from build123d import *

# Parameters (mm, degrees)
SKETCH2_W               = 20
SKETCH2_H               = 49.91
BOSS_EXTRUDE1_DEPTH     = 44.5
CUT_EXTRUDE3_DEPTH      = 68.611079713
CUT_EXTRUDE5_DEPTH      = 55.799653512
CUT_EXTRUDE5_DEPTH_BACK = 55.799653512
SKETCH8_R               = 2.6
SKETCH8_R_2             = 2.35
SKETCH9_R               = 2.1
CUT_EXTRUDE6_DEPTH      = 6.6
SKETCH9_3_R             = 3.35
CUT_EXTRUDE7_DEPTH      = 0.8
CUT_EXTRUDE8_START      = -0.8
SKETCH11_R              = 3.35
CUT_EXTRUDE8_DEPTH      = 0.8
SKETCH12_W              = 6.8
SKETCH12_H              = 15.77
CUT_EXTRUDE9_DEPTH      = 15


with BuildPart() as part:
    # Sketch2 → Boss-Extrude1 (new body)
    with BuildSketch(Plane(origin=(0, 0, 0), x_dir=(1, 0, 0), z_dir=(0, 1, 0))):
        Rectangle(SKETCH2_W, SKETCH2_H)
    extrude(amount=BOSS_EXTRUDE1_DEPTH)

    # Sketch3 → Cut-Extrude3 (cut, through all)
    with BuildSketch(Plane.XY.offset(24.955)):
        Polygon((3.4, 44.5), (-3.4, 44.5), (-3.4, 23.020172412), (-2.5, 23.020172412), (-2.5, 7.250172412), (2.5, 7.250172412), (2.5, 23.020172412), (3.4, 23.020172412), align=None)
    extrude(amount=-CUT_EXTRUDE3_DEPTH, mode=Mode.SUBTRACT)

    # Sketch8 → Cut-Extrude5 (cut, two sides: drawn at the far end of the back side and taken through both)
    with BuildSketch(Plane.ZY.offset(10).offset(-CUT_EXTRUDE5_DEPTH_BACK)):
        with Locations((-12.865, 32.41)):
            Circle(SKETCH8_R)
        with Locations((12.955, 32.41)):
            Circle(SKETCH8_R_2)
    extrude(amount=CUT_EXTRUDE5_DEPTH + CUT_EXTRUDE5_DEPTH_BACK, mode=Mode.SUBTRACT)

    # Sketch9 → Cut-Extrude6 (cut)
    with BuildSketch(Plane(origin=(10, 0, 0), x_dir=(0, 0, -1), z_dir=(1, 0, 0))):
        with Locations((-6.045, 21.485172412)):
            Circle(SKETCH9_R)
        with Locations((-6.045, 8.785172412)):
            Circle(SKETCH9_R)
    extrude(amount=-CUT_EXTRUDE6_DEPTH, mode=Mode.SUBTRACT)

    # Sketch9_3 → Cut-Extrude7 (cut)
    with BuildSketch(Plane(origin=(10, 0, 0), x_dir=(0, 0, -1), z_dir=(1, 0, 0))):
        with Locations((-6.045, 21.485172412)):
            Circle(SKETCH9_3_R)
        with Locations((-6.045, 8.785172412)):
            Circle(SKETCH9_3_R)
    extrude(amount=-CUT_EXTRUDE7_DEPTH, mode=Mode.SUBTRACT)

    # Sketch11 → Cut-Extrude8 (cut)
    with BuildSketch(Plane.ZY.offset(-3.4).offset(CUT_EXTRUDE8_START)):
        with Locations(Location((6.045, 21.485172412, 0), (0, 0, 180))):
            Circle(SKETCH11_R)
        with Locations(Location((6.045, 8.785172412, 0), (0, 0, 180))):
            Circle(SKETCH11_R)
    extrude(amount=CUT_EXTRUDE8_DEPTH, mode=Mode.SUBTRACT)

    # Sketch12 → Cut-Extrude9 (cut)
    with BuildSketch(Plane(origin=(0, 0, -24.955), x_dir=(-1, 0, 0), z_dir=(0, 0, -1))):
        with Locations((0, 15.135172412)):
            Rectangle(SKETCH12_W, SKETCH12_H)
    extrude(amount=-CUT_EXTRUDE9_DEPTH, mode=Mode.SUBTRACT)


solid = part.part
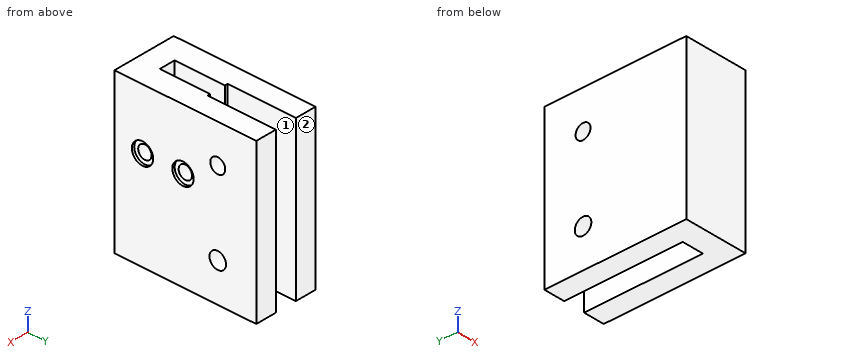
Check sheet for the modelled part. Datum: model origin and axes. Units: mm. Face numbers are marked on the shaded views. A direction names the side the tool comes from. Give positions to 0.01 mm unless a question says otherwise; leave off trailing zeros. Order: outer loops, then holes, each group sorted by start corner. A loop starts at its lowest first (then second) coordinate and runs counter-clockwise, first axis right, second up. Notation, with made-up numbers: M -9.5,22.25 L 23.5,22.25 A20 ccw 23.5,30.25 Z; hole C 83.25,56 d1. An arc over 180 degrees is marked long. Answer as CSV lines item,"result". Start each with the question number.
Item 1: Gauge pin test, flat ends, axial feed: P1, Ø7.5, axis at y = 9, z = 6, coming from the +X side; P2, Ø3.5, axis at x = 0, z = 3, coming from the +Y side; P3, Ø4, axis at y = 21.5, z = 6.5, coming from the +X side; P4, Ø0.7, axis at x = 3, y = 13, coming from the -Z side (3 decimals). Record the tip position at first contact, or that the pin passes through.
Item 2: Cross-section at B-B on z = -20. Enter the section's corners in (x, y).
Item 3: Cross-section at C-C on x = 6. Enter the section's corners in (y, z) (3 decimals).
Item 4: Tool access check on the marked faces 1 and 2. Record the directions out of +Z, -Z, +X, -X, +Y, -Y that give a thin tool (end or side, any length) a straight path to the whole face; none if there is none.
Item 5: Cross-section at D-D on y = 17. Enter the section's corners in (x, z) (3 decimals), plus the area to 3 significant figures.
Item 6: Cross-section at A-A on y = 28.5. Enter the section's corners in (x, z) (3 decimals).
Item 7: Thickness scan on line 1 (Z direction, x = 7.5, y = 32.41) (3 decimals); line 2 (X direction, y = 30, z = -20.5); line 3 (X direction, y = 18, z = 4). Record the ranges inside material, lowest first. Write a range as [from, to].
Established:
1,P1,"stops at x = 10"
1,P2,"stops at y = 7.25"
1,P3,"stops at x = 9.2"
1,P4,"stops at z = -9.955"
2,outline,"M -10,0 L 10,0 L 10,44.5 L 3.4,44.5 L 3.4,7.25 L -3.4,7.25 L -3.4,44.5 L -10,44.5 Z"
3,outline,"M 0,-24.955 L 44.5,-24.955 L 44.5,24.955 L 0,24.955 Z; hole C 8.785,6.045 d4.2; hole C 21.485,6.045 d4.2; hole C 32.41,-12.865 d5.2; hole C 32.41,12.955 d4.7"
4,face 1,"-Z, +Y"
4,face 2,"+Z, -Z, +X, -X, +Y"
5,outline,"M -10,-24.955 L -3.4,-24.955 L -3.4,-9.955 L -2.5,-9.955 L -2.5,24.955 L -10,24.955 Z; M 2.5,-9.955 L 3.4,-9.955 L 3.4,-24.955 L 10,-24.955 L 10,24.955 L 2.5,24.955 Z"
5,area,"722 mm^2"
6,outline,"M -10,-24.955 L -3.4,-24.955 L -3.4,24.955 L -10,24.955 Z; M 3.4,-24.955 L 10,-24.955 L 10,24.955 L 3.4,24.955 Z"
7,line 1,"z = [-24.955, -15.465], [-10.265, 10.605], [15.305, 24.955]"
7,line 2,"x = [-10, -3.4], [3.4, 10]"
7,line 3,"x = [-10, -2.5], [2.5, 10]"
